Input: part model. Units: mm. Frame: model coordinates. Face numbers are marked on the shaded views. A direction names the side the tool comes from. Coordinates: 2 decimals unless noted, no trailing zeros. Loops run counter-clockwise (first coordinate to the right, second up) from the corner with the lowest first, then second, coordinate; pieces in that order, holes last.
Item 1: Section A-A on y = 32. Return loops of the section in (x, z), and give its area (3 significant figures).
Item 2: Section B-B on z = 3. Return loops of the section in (x, y), and give its area (3 significant figures).
Item 3: Pull-direction query (Z, two-part tool) for the marked faces 6, 7, 8 and 9; classes: released by +Z, released by -Z, zero draft, split by the parting line, or undercut.
Item 4: Reachability of the marked faces 1, 2, 3, 4 and 5 from +Z, -Z, +X, -X, +Y, -Y: full face, straight path, thin tool, end or side. Return the list, or none.
Item 5: Ray query, line 1 along Y through (x, z) = (29.5, 8); line 2 along Y through (x, z) = (35.75, 2.4); line 3 along X through (y, z) = (10, 1.5). Return the intervals inside material, ascending.
Item 6: Contact query for flat-ended pins moving along their axis: P1, Ø8, axis at y = 23, z = 4.5, coming from the +X side; P2, Ø8, axis at x = 7, y = 20, coming from the +Z side; P3, Ø1.5, axis at y = 7, z = 17.5, coming from the -X side; P4, Ø0.7, axis at y = -36.5, z = 14.5, coming from the -X side. Output: stop coordinate, or through.
Item 7: Section C-C on x = 30. Give the number of separate pieces and of enclosed holes in the cut face, and give its area (3 significant figures).
Item 8: Section D-D on x = 5. Return loops of the section in (y, z).
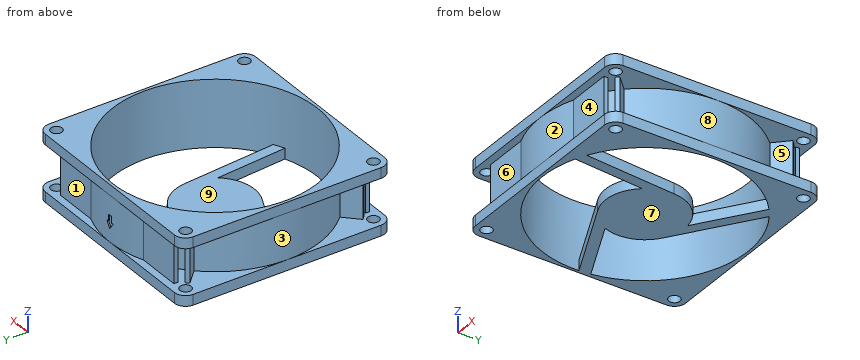
```python
from build123d import *

# Parameters (mm, degrees)
SKETCH_BODY_R                       = 39
BODY_DEPTH                          = 25.4
SKETCH_CUT_BODY_W                   = 17.4
SKETCH_CUT_BODY_H                   = 14.808134855
REINFORCMENT_STRIP_REACH            = 64.009
CIRPATTERN_REINFORCMENT_STRIP_COUNT = 4
SKETCH_FIXING_HOLE_R                = 2.15
FIXING_HOLE_DEPTH                   = 63.009354133
CIRPATTERN_FIXING_HOLE_COUNT        = 4
BONE_DEPTH                          = 4
CIRPATTERN_BONE_COUNT               = 3
REINFORCMENT_PLATES_REACH           = 64.009
SKETCH_FIXING_PLATE_FAN_R           = 15
FIXING_PLATE_FAN_DEPTH              = 4
AIR_EXHAUST_DEPTH                   = 93.549500269


with BuildPart() as part:
    # Sketch-Body → Body (new body)
    with BuildSketch(Plane.XY):
        with BuildLine():
            Line((-35.75, -40), (35.75, -40))
            ThreePointArc((35.75, -40), (38.75520382, -38.75520382), (40, -35.75))
            Line((40, -35.75), (40, 35.75))
            ThreePointArc((40, 35.75), (38.75520382, 38.75520382), (35.75, 40))
            Line((35.75, 40), (-35.75, 40))
            ThreePointArc((-35.75, 40), (-38.75520382, 38.75520382), (-40, 35.75))
            Line((-40, 35.75), (-40, -35.75))
            ThreePointArc((-40, -35.75), (-38.75520382, -38.75520382), (-35.75, -40))
        make_face()
        Circle(SKETCH_BODY_R, mode=Mode.SUBTRACT)
    extrude(amount=BODY_DEPTH)

    # Sketch-Cut-Body → Cut-Body (revolve, cut)
    with BuildSketch(Plane(origin=(0, 0, 0), x_dir=(0, 0, -1), z_dir=(1, 0, 0)), mode=Mode.PRIVATE) as cut_body_sk:
        with Locations((-12.7, 47.404067428)):
            Rectangle(SKETCH_CUT_BODY_W, SKETCH_CUT_BODY_H)
    revolve(cut_body_sk.sketch.rotate(Axis((0, 0, 25.4), (0, 0, -1)), 180), axis=Axis((0, 0, 25.4), (0, 0, -1)), mode=Mode.SUBTRACT)

    # Sketch-Reinforcment-Strip → Reinforcment-Strip (add, up to next)
    with BuildSketch(Plane.XY, mode=Mode.PRIVATE) as reinforcment_strip_sk1:
        with BuildLine():
            Line((28.801838692, 27.757054743), (33.991972605, 32.947188656))
            Line((33.991972605, 32.947188656), (32.947188656, 33.991972605))
            Line((32.947188656, 33.991972605), (27.757054743, 28.801838692))
            ThreePointArc((27.757054743, 28.801838692), (28.284271247, 28.284271247), (28.801838692, 27.757054743))
        make_face()
    reinforcment_strip_tool1 = extrude(reinforcment_strip_sk1.sketch, amount=REINFORCMENT_STRIP_REACH, mode=Mode.PRIVATE) - part.part
    reinforcment_strip = reinforcment_strip_tool1.solids().sort_by_distance((30.876122, 30.876122, 0))[0]
    add(reinforcment_strip)

    # CirPattern-Reinforcment-Strip: Reinforcment-Strip ×4 about axis
    cirpattern_reinforcment_strip_axis = Axis((0, 0, 0), (0, 0, 1))
    for i in range(1, CIRPATTERN_REINFORCMENT_STRIP_COUNT):
        add(reinforcment_strip.rotate(cirpattern_reinforcment_strip_axis, i * 360 / CIRPATTERN_REINFORCMENT_STRIP_COUNT))

    # Sketch-Fixing-Hole → Fixing-Hole (cut, through all)
    with BuildSketch(Plane.XY):
        with Locations(Location((35.75, 35.75, 0), (0, 0, 90))):
            Circle(SKETCH_FIXING_HOLE_R)
    fixing_hole = extrude(amount=FIXING_HOLE_DEPTH, mode=Mode.SUBTRACT)

    # CirPattern-Fixing-Hole: Fixing-Hole ×4 about axis
    cirpattern_fixing_hole_axis = Axis((0, 0, 0), (0, 0, 1))
    for i in range(1, CIRPATTERN_FIXING_HOLE_COUNT):
        add(fixing_hole.rotate(cirpattern_fixing_hole_axis, i * 360 / CIRPATTERN_FIXING_HOLE_COUNT), mode=Mode.SUBTRACT)

    # Sketch-Bone → Bone (add)
    with BuildSketch(Plane.XY):
        with BuildLine():
            Line((14.980149429, 0.771442214), (18.07129405, -34.560502476))
            ThreePointArc((18.07129405, -34.560502476), (16.164518677, -35.492370109), (14.209874971, -36.319133433))
            Line((14.209874971, -36.319133433), (11.838280423, -9.211683702))
            ThreePointArc((11.838280423, -9.211683702), (14.308135647, -4.503027238), (14.980149429, 0.771442214))
        make_face()
    bone = extrude(amount=BONE_DEPTH)

    # CirPattern-Bone: Bone ×3 about axis
    cirpattern_bone_axis = Axis((0, 0, 0), (0, 0, 1))
    for i in range(1, CIRPATTERN_BONE_COUNT):
        add(bone.rotate(cirpattern_bone_axis, i * 360 / CIRPATTERN_BONE_COUNT))

    # Sketch3 → Reinforcment-Plates (add, up to next)
    with BuildSketch(Plane.XY, mode=Mode.PRIVATE) as reinforcment_plates_sk1:
        with BuildLine():
            Line((14.632487739, 37.227547631), (31.45, 37.227547631))
            Line((31.45, 37.227547631), (31.45, 35.75))
            Line((31.45, 35.75), (17.942616866, 35.75))
            ThreePointArc((17.942616866, 35.75), (16.304298413, 36.526289892), (14.632487739, 37.227547631))
        make_face()
    reinforcment_plates_tool1 = extrude(reinforcment_plates_sk1.sketch, amount=REINFORCMENT_PLATES_REACH, mode=Mode.PRIVATE) - part.part
    # Sketch3 → Reinforcment-Plates (add, up to next)
    with BuildSketch(Plane.XY, mode=Mode.PRIVATE) as reinforcment_plates_sk2:
        with BuildLine():
            Line((-31.45, 35.75), (-17.942616866, 35.75))
            ThreePointArc((-17.942616866, 35.75), (-16.304298413, 36.526289892), (-14.632487739, 37.227547631))
            Line((-14.632487739, 37.227547631), (-31.45, 37.227547631))
            Line((-31.45, 37.227547631), (-31.45, 35.75))
        make_face()
    reinforcment_plates_tool2 = extrude(reinforcment_plates_sk2.sketch, amount=REINFORCMENT_PLATES_REACH, mode=Mode.PRIVATE) - part.part
    # Sketch3 → Reinforcment-Plates (add, up to next)
    with BuildSketch(Plane.XY, mode=Mode.PRIVATE) as reinforcment_plates_sk3:
        with BuildLine():
            Line((-31.45, -37.227547631), (-31.45, -35.75))
            Line((-31.45, -35.75), (-17.942616866, -35.75))
            ThreePointArc((-17.942616866, -35.75), (-16.304298413, -36.526289892), (-14.632487739, -37.227547631))
            Line((-14.632487739, -37.227547631), (-31.45, -37.227547631))
        make_face()
    reinforcment_plates_tool3 = extrude(reinforcment_plates_sk3.sketch, amount=REINFORCMENT_PLATES_REACH, mode=Mode.PRIVATE) - part.part
    # Sketch3 → Reinforcment-Plates (add, up to next)
    with BuildSketch(Plane.XY, mode=Mode.PRIVATE) as reinforcment_plates_sk4:
        with BuildLine():
            Line((14.632487739, -37.227547631), (31.45, -37.227547631))
            Line((31.45, -37.227547631), (31.45, -35.75))
            Line((31.45, -35.75), (17.942616866, -35.75))
            ThreePointArc((17.942616866, -35.75), (16.304298413, -36.526289892), (14.632487739, -37.227547631))
        make_face()
    reinforcment_plates_tool4 = extrude(reinforcment_plates_sk4.sketch, amount=REINFORCMENT_PLATES_REACH, mode=Mode.PRIVATE) - part.part
    add(reinforcment_plates_tool1.solids().sort_by_distance((23.872253, 36.515707, 0))[0])
    add(reinforcment_plates_tool2.solids().sort_by_distance((-23.872253, 36.515707, 0))[0])
    add(reinforcment_plates_tool3.solids().sort_by_distance((-23.872253, -36.515707, 0))[0])
    add(reinforcment_plates_tool4.solids().sort_by_distance((23.872253, -36.515707, 0))[0])

    # Sketch-Fixing-Plate-Fan → Fixing-Plate-Fan (add)
    with BuildSketch(Plane.XY):
        Circle(SKETCH_FIXING_PLATE_FAN_R)
    extrude(amount=FIXING_PLATE_FAN_DEPTH)

    # Sketch5 → Air-Exhaust (cut, through all)
    with BuildSketch(Plane(origin=(0, 39.5, 0), x_dir=(-1, 0, 0), z_dir=(0, 1, 0))):
        Polygon((0.881634904, 14), (-0.881634904, 14), (-0.881634904, 11.5), (-1.750518846, 11.5), (0, 9), (1.750518846, 11.5), (0.881634904, 11.5), align=None)
    extrude(amount=AIR_EXHAUST_DEPTH, mode=Mode.SUBTRACT)


solid = part.part
```
Results found:
1. outline: (-40, 0) - (-22.29, 0) - (-22.29, 25.4) - (-40, 25.4) - (-40, 21.4) - (-33.04, 21.4) - (-33.04, 4) - (-40, 4) - close; (19.57, 0) - (40, 0) - (40, 4) - (33.04, 4) - (33.04, 21.4) - (40, 21.4) - (40, 25.4) - (22.29, 25.4) - (22.29, 4) - (19.57, 4) - close; hole (-30.96, 4) - (-24, 4) - (-24, 21.4) - (-30.96, 21.4) - close; hole (24, 4) - (30.96, 4) - (30.96, 21.4) - (24, 21.4) - close
1. area: 426 mm2
2. outline: (-40, -35.75) arc R4.25 ccw to (-35.75, -40) - (35.75, -40) arc R4.25 ccw to (40, -35.75) - (40, 35.75) arc R4.25 ccw to (35.75, 40) - (-35.75, 40) arc R4.25 ccw to (-40, 35.75) - close; hole (-38.97, 1.63) arc R39 ccw to (14.21, -36.32) - (11.84, -9.21) arc R15 cw to (-6.82, -13.36) - close; hole (-38.56, 5.85) - (-13.9, -5.65) arc R15 cw to (-8.16, 12.59) - (20.89, 32.93) arc R39 ccw to start; hole circle Ø4.3 at (-35.75, -35.75); hole circle Ø4.3 at (-35.75, 35.75); hole (2.06, 14.86) arc R15 cw to (14.98, 0.77) - (18.07, -34.56) arc R39 ccw to (24.35, 30.47) - close; hole circle Ø4.3 at (35.75, -35.75); hole circle Ø4.3 at (35.75, 35.75)
2. area: 2,610 mm2
3. face 6: undercut
3. face 7: released by -Z
3. face 8: undercut
3. face 9: released by +Z
4. face 1: +X, +Y
4. face 2: -Y
4. face 3: -X
4. face 4: +X, -Y
4. face 5: +X
5. line 1: y = -37.23 to -35.75, -30.54 to -28.46, -27.01 to -25.51, 25.51 to 27.01, 28.46 to 30.54, 35.75 to 37.23
5. line 2: y = -40 to -37.9, -33.6 to -15.59, 15.59 to 33.6, 37.9 to 40
5. line 3: x = -40 to -37.7, -11.18 to 11.18, 37.7 to 40
6. P1: stops at x = 40
6. P2: stops at z = 4
6. P3: stops at x = -39.51
6. P4: stops at x = -31.45
7. separate pieces: 2
7. enclosed holes: 4
7. area: 419 mm2
8. outline: (-40, 0) - (-38.68, 0) - (-38.68, 25.4) - (-40, 25.4) - (-40, 21.4) - (-39.69, 21.4) - (-39.69, 4) - (-40, 4) - close; (-14.14, 0) - (14.14, 0) - (14.14, 4) - (-14.14, 4) - close; (16.92, 0) - (21.8, 0) - (21.8, 4) - (16.92, 4) - close; (38.68, 0) - (40, 0) - (40, 4) - (39.69, 4) - (39.69, 21.4) - (40, 21.4) - (40, 25.4) - (38.68, 25.4) - close
